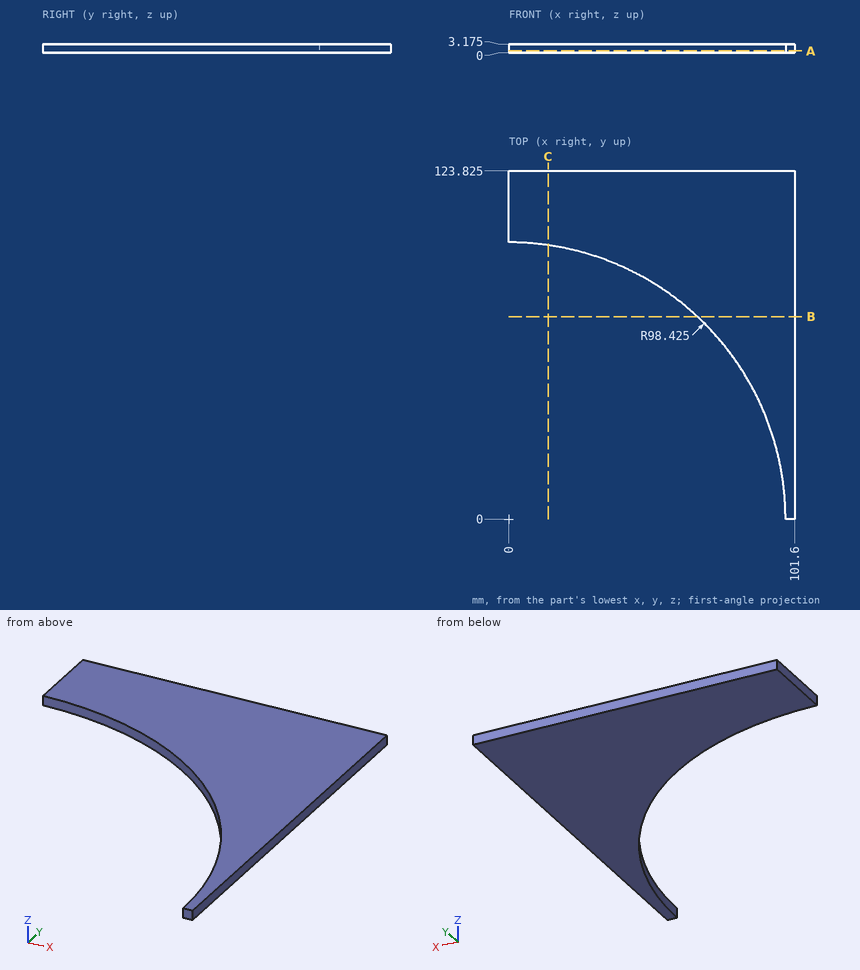
Job drawing, mm, ordinate dimensions from the low corner. One solid piece. Coordinates: 2 decimals unless noted, no trailing zeros. Order: outer loops, then holes, each group sorted by start corner. A loop starts at its lowest first (then second) coordinate and runs counter-clockwise, first axis right, second up. Notation, with made-up numbers: M 3,14.25 L 37,14.25 A27 ccw 37,43.25 Z; hole C 81,-33 d9. An arc over 180 degrees is marked long. One line per question, with ' | ' between items.
Q1. Drill centre lines: line 1 (X direction, y = 68, z = 0.5); line 2 (X direction, y = 51.5, z = 1.9); line 3 (Y direction, x = 63, z = 2.15) (3 decimals). Where is each one in solid material? Low to high.
A:
line 1: x = 71.16 to 101.6 | line 2: x = 83.88 to 101.6 | line 3: y = 75.621 to 123.825
Q2. Pin check, flat tip, straight feed: P1, Ø1.5, axis at x = 26.5, z = 2.5, coming from the -Y side. Stop position of the tip, or through.
A:
P1: stops at y = 94.58
Q3. Slice it at C-C (x = 14). Give the cut face in (y, z) (3 decimals).
A:
outline: M 97.424,0 L 123.825,0 L 123.825,3.175 L 97.424,3.175 Z
Q4. Slice it at B-B (y = 72). Give the cut face in (x, z) (3 decimals).
A:
outline: M 67.108,0 L 101.6,0 L 101.6,3.175 L 67.108,3.175 Z
Q5. Slice it at A-A (z = 0.7). Give the cut face in (x, y) (3 decimals).
A:
outline: M 0,98.425 A98.425 cw 98.425,0 L 101.6,0 L 101.6,123.825 L 0,123.825 Z
